Job drawing, mm, ordinate dimensions from the low corner. One solid piece. A direction names the side the tool comes from. Give positions to 0.01 mm unless a question says otherwise; leave off trailing zeros. Order: outer loops, then holes, each group sorted by start corner. A loop starts at its lowest first (then second) coordinate and runs counter-clockwise, first axis right, second up.
Item 1: Band-saw the part on A-A on x = 14. Give the cut face in (y, z), plus the area to 3 significant figures.
Item 2: Flat gauge pins, fed straight in: P1, Ø1, axis at x = 16, z = 4, coming from the -Y side; P2, Ø2, axis at x = 57.5, z = 3.5, coming from the +Y side; P3, Ø2.5, axis at x = 56.5, z = 3, coming from the +Y side. Where does each tip first touch, or does it go through?
Item 3: Which spindle directions (+Z, -Z, +X, -X, +Y, -Y) get a long thin tool onto all of the face, cutting with end or side? Do the marked faces 4 and 5. Say none if no direction does.
Item 4: Wall check: L1, parallel to X at y = 8.5, z = 1.5 (1 decimal); L2, parallel to Y at x = 39.5, z = 0.4 (1 decimal); L3, parallel to Y at x = 56, z = 4.5. Give the ranges that are in metal, low to high.
Item 5: Band-saw the part on C-C on z = 2.3. Give the cut face in (x, y), plus the area to 3 significant figures.
Item 6: Two-plate mould, pull along X, no slides. Class the marked faces 1, 2 and 3: released by +X, released by -X, zero draft, split by the parting line, or undercut.
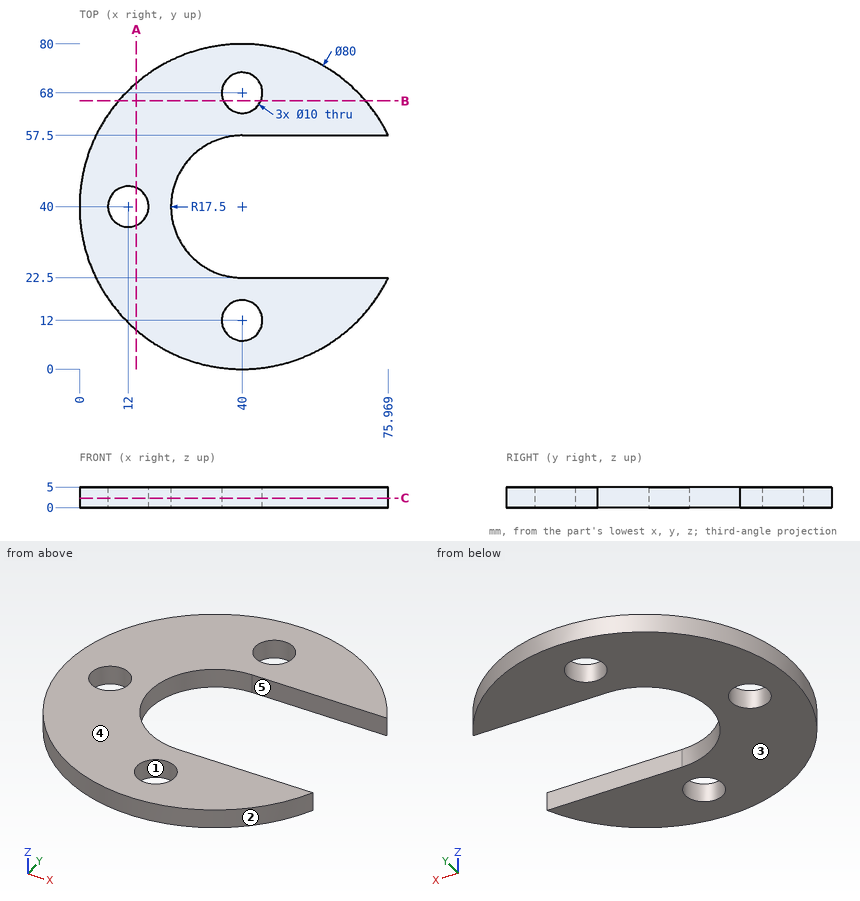
The answers:
1. outline: (9.6, 0) - (35.42, 0) - (35.42, 5) - (9.6, 5) - close; (44.58, 0) - (70.4, 0) - (70.4, 5) - (44.58, 5) - close
1. area: 258 mm2
2. P1: stops at y = 7.63
2. P2: stops at y = 76.44
2. P3: stops at y = 76.98
3. face 4: +Z, +X, -X, +Y, -Y
3. face 5: +Z, -Z, +X
4. L1: x = 15.3 to 36.4, 43.6 to 64.7
4. L2: y = 0 to 7, 17 to 22.5, 57.5 to 63, 73 to 80
4. L3: y = 3.34 to 22.5, 57.5 to 76.66
5. outline: (40, 22.5) arc R17.5 cw to (40, 57.5) - (75.97, 57.5) arc R40 ccw (long way) to (75.97, 22.5) - close; hole circle Ø10 at (12, 40); hole circle Ø10 at (40, 12); hole circle Ø10 at (40, 68)
5. area: 2,960 mm2
6. face 1: undercut
6. face 2: split by the parting line
6. face 3: zero draft
